from build123d import *

# Parameters (mm, degrees)
SKETCH_R        = 43
SKETCH_R_2      = 41
PAD_DEPTH       = 5
SKETCH001_R     = 43.5
SKETCH001_R_2   = 34
PAD001_DEPTH    = 1
SKETCH002_R     = 40
SKETCH002_R_2   = 37.7
PAD002_DEPTH    = 10
CHAMFER_SIZE    = 1
CHAMFER001_SIZE = 1


with BuildPart() as part:
    # Sketch → Pad (new body)
    with BuildSketch(Plane.XY):
        Circle(SKETCH_R)
        Circle(SKETCH_R_2, mode=Mode.SUBTRACT)
    extrude(amount=PAD_DEPTH)

    # Sketch001 (on Face4 of Pad) → Pad001 (join)
    with BuildSketch(Plane.XY.offset(5)):
        Circle(SKETCH001_R)
        Circle(SKETCH001_R_2, mode=Mode.SUBTRACT)
    extrude(amount=PAD001_DEPTH)

    # Sketch002 (on Face3 of Pad001) → Pad002 (join)
    with BuildSketch(Plane.XY.offset(6)):
        Circle(SKETCH002_R)
        Circle(SKETCH002_R_2, mode=Mode.SUBTRACT)
    extrude(amount=PAD002_DEPTH)

    # Chamfer
    chamfer_edges = [part.edges().sort_by_distance(p)[0] for p in [
        (-40, 0, 16),
    ]]
    chamfer(chamfer_edges, length=CHAMFER_SIZE)

    # Chamfer001
    chamfer001_edges = [part.edges().sort_by_distance(p)[0] for p in [
        (-41, 0, 0),
    ]]
    chamfer(chamfer001_edges, length=CHAMFER001_SIZE)


solid = part.part
Source: CAD feature listing. Evaluate the final solid. Frame: model axes, mm. A direction names the side the tool comes from. Give positions to 0.01 mm unless a question says otherwise; leave off trailing zeros. Order: outer loops, then holes, each group sorted by start corner. A loop starts at its lowest first (then second) coordinate and runs counter-clockwise, first axis right, second up. Notation, with made-up numbers: (40.5, 25) -> (83.5, 25) arc R18 cw to (83.5, 38) -> close; hole circle Ø11 at (14, 59). An arc over 180 degrees is marked (long way). Write item = value, one per line.
Item 1: Mould query, pull axis Y, two halves, no side actions, for faces 1 (the face through (38, -13, 6)), 2 (the face through (-8.67, -39.05, 10.44)), 3 (the face through (-6, 34, 6)). Classes: +Y half, -Y half, draft (parallel to the pull), parting line (faces both ways), or undercut.
Check result:
face_1 = draft
face_2 = parting line
face_3 = undercut
Item 2: Contact query for flat-ended pins moving along their axis: pin 1 (1 mm diameter, centred on x = 29.5, y = -18.5, fed in from +Z); pin 2 (4 mm diameter, centred on x = -26, y = -15, fed in from +Z); pin 3 (24.5 mm diameter, centred on x = -19.5, y = -18.5, fed in from -Z); pin 4 (3 mm diameter, centred on x = -8, z = 4.5, fed in from +Y). Output: stop coordinate, or through.
Check result:
pin_1 = 6
pin_2 = through
pin_3 = 5
pin_4 = 43
Item 3: Section query C-C (z = 9.25). Output: boundary loops of the cut face in (x, y).
Check result:
outline = circle Ø80 at (0, 0); hole circle Ø75.4 at (0, 0)
Item 4: Set-up query: faces 4 (the face through (-8.173, -36.804, 10.93)), 5 (the face through (-42, 10, 5)), 6 (the face through (18.28, 28.67, 5.49)). Return all of +Z, -Z, +X, -X, +Y, -Y with unobstructed straight access to the full face (end or side cutting, diameter ignored); none if empty.
Check result:
face_4 = +Z
face_5 = -Z
face_6 = +Z, -Z
Item 5: Section query D-D (z = 2.25). Output: boundary loops of the cut face in (x, y).
Check result:
outline = circle Ø86 at (0, 0); hole circle Ø82 at (0, 0)
Item 6: Section query A-A (x = 0). Output: boundary loops of the cut face in (y, z), then the cut area to 3 significant figures.
Check result:
outline = (-43.5, 5) -> (-43, 5) -> (-43, 0) -> (-42, 0) -> (-41, 1) -> (-41, 5) -> (-34, 5) -> (-34, 6) -> (-37.7, 6) -> (-37.7, 16) -> (-39, 16) -> (-40, 15) -> (-40, 6) -> (-43.5, 6) -> close; (34, 5) -> (41, 5) -> (41, 1) -> (42, 0) -> (43, 0) -> (43, 5) -> (43.5, 5) -> (43.5, 6) -> (40, 6) -> (40, 15) -> (39, 16) -> (37.7, 16) -> (37.7, 6) -> (34, 6) -> close
area = 83.0 mm²
Item 7: Ray query, probe 1 along Y at (x, z) = (0, 5.5); probe 2 along Y at (x, z) = (0, 10.5); probe 3 along X at (y, z) = (6, 6.25). Return the intervals inside material, ascending.
Check result:
probe_1 = -43.5 to -34, 34 to 43.5
probe_2 = -40 to -37.7, 37.7 to 40
probe_3 = -39.55 to -37.22, 37.22 to 39.55
